The model under review builds one solid part; all positions refer to its coordinate system, in mm. Give positions to 0.01 mm unless a question says otherwise; leave off trailing zeros. Order: outer loops, then holes, each group sorted by start corner. A loop starts at its lowest first (then second) coordinate and runs counter-clockwise, first axis right, second up. Notation, with made-up numbers: (26, -22) - (48, -22) arc R20 ccw to (48, -7) - close; hole circle Ø1 at (-3.5, 6.25). An arc over 180 degrees is marked (long way). Put each result on its own line as item: value.
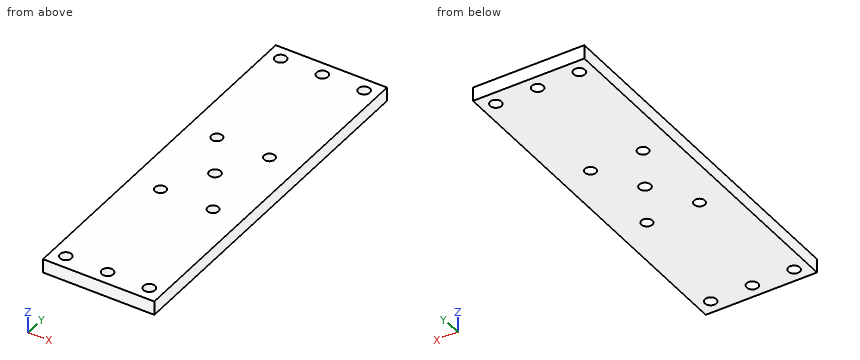
```python
from build123d import *

# Parameters (mm, degrees)
F0_W     = 50.8
F0_H     = 6.35
F1_DEPTH = 165.1
F2_R     = 2.6162
F2_R_2   = 2.5019
F3_DEPTH = 6.351


with BuildPart() as f1:
    # F0 (on Front) → F1 (new body)
    with BuildSketch(Plane.XZ):
        Rectangle(F0_W, F0_H)
    extrude(amount=F1_DEPTH)

    # F2 (on face) → F3 (cut, through all)
    with BuildSketch(Plane.XY.offset(3.175)):
        with Locations((0, -158.75)):
            Circle(F2_R)
        with Locations((0, -6.35)):
            Circle(F2_R)
        with Locations((-12.0015, -102.5525)):
            Circle(F2_R_2)
        with Locations((12.0015, -102.5525)):
            Circle(F2_R_2)
        with Locations((12.0015, -62.5475)):
            Circle(F2_R_2)
        with Locations((-12.0015, -62.5475)):
            Circle(F2_R_2)
        with Locations((0, -82.55)):
            Circle(F2_R)
        with Locations((-19.05, -158.75)):
            Circle(F2_R)
        with Locations((19.05, -158.75)):
            Circle(F2_R)
        with Locations((-19.05, -6.35)):
            Circle(F2_R)
        with Locations((19.05, -6.35)):
            Circle(F2_R)
    extrude(amount=-F3_DEPTH, mode=Mode.SUBTRACT)


solid = f1.part
```
(1) Take a section at C-C, the plane y = -6.35. Write out the cut boundary in (x, z) (3 decimals).
The answers:
outline: (-25.4, -3.175) - (-21.666, -3.175) - (-21.666, 3.175) - (-25.4, 3.175) - close; (-16.434, -3.175) - (-2.616, -3.175) - (-2.616, 3.175) - (-16.434, 3.175) - close; (2.616, -3.175) - (16.434, -3.175) - (16.434, 3.175) - (2.616, 3.175) - close; (21.666, -3.175) - (25.4, -3.175) - (25.4, 3.175) - (21.666, 3.175) - close
(2) Clearance check with a flat-ended pin moving along its axis: pin 1 Ø4.5 at (x, y) = (0, -82.55) entering from -Z. State where the tip first meets the part, or that it passes through.
The answers:
pin 1: through
(3) Take a section at A-A, the plane x = -19.05. Write out the cut boundary in (y, z) (3 decimals).
The answers:
outline: (-165.1, -3.175) - (-161.366, -3.175) - (-161.366, 3.175) - (-165.1, 3.175) - close; (-156.134, -3.175) - (-8.966, -3.175) - (-8.966, 3.175) - (-156.134, 3.175) - close; (-3.734, -3.175) - (0, -3.175) - (0, 3.175) - (-3.734, 3.175) - close
(4) Take a section at B-B, the plane y = -82.55. Write out the cut boundary in (x, z) (3 decimals).
The answers:
outline: (-25.4, -3.175) - (-2.616, -3.175) - (-2.616, 3.175) - (-25.4, 3.175) - close; (2.616, -3.175) - (25.4, -3.175) - (25.4, 3.175) - (2.616, 3.175) - close
(5) Wall thickness on L1, parallel to Y at x = -19.05, z = 0; L2, parallel to Y at x = 0, z = 1.5; L3, parallel to X at y = -102.5, z = -0.5: over which ranges is each line inside the solid? List them lowest first.
The answers:
L1: -165.1 to -161.37, -156.13 to -8.97, -3.73 to 0
L2: -165.1 to -161.37, -156.13 to -85.17, -79.93 to -8.97, -3.73 to 0
L3: -25.4 to -14.5, -9.5 to 9.5, 14.5 to 25.4
(6) Take a section at D-D, the plane x = 0. Write out the cut boundary in (y, z) (3 decimals).
The answers:
outline: (-165.1, -3.175) - (-161.366, -3.175) - (-161.366, 3.175) - (-165.1, 3.175) - close; (-156.134, -3.175) - (-85.166, -3.175) - (-85.166, 3.175) - (-156.134, 3.175) - close; (-79.934, -3.175) - (-8.966, -3.175) - (-8.966, 3.175) - (-79.934, 3.175) - close; (-3.734, -3.175) - (0, -3.175) - (0, 3.175) - (-3.734, 3.175) - close
